Build history of the part. All positions in model axes, mm. Face numbers are marked on the shaded views. Give positions to 0.01 mm unless a question says otherwise; leave off trailing zeros. Order: outer loops, then holes, each group sorted by start corner. A loop starts at its lowest first (then second) coordinate and runs counter-clockwise, first axis right, second up. Notation, with made-up numbers: M 57.25,14.5 L 62.25,14.5 A16 ccw 62.25,41.5 Z; hole C 36,-4.75 d2. An arc over 180 degrees is marked long. One line per item, written item: value. Start each with the question number.
Autodesk Inventor part; units mm, degrees
ref_plane "YZ Plane" through (0, 0, 0) normal (1, 0, 0) x (0, 1, 0)
ref_plane "XZ Plane" through (0, 0, 0) normal (0, 1, 0) x (-1, 0, 0)
ref_plane "XY Plane" through (0, 0, 0) normal (0, 0, 1) x (1, 0, 0)
sketch "Sketch1" plane through (0, 0, 0) normal (0, 0, 1) x (1, 0, 0)
  circle A0 centre (0, 0) radius 3.9688
  dimension "d0" = 7.9375
extrude "Extrusion1" add sketch "Sketch1" along normal blind 78
thread "Thread1"
sketch "Sketch2" plane through (0, 0, 78) normal (0, 0, 1) x (1, 0, 0)
  circle A0 centre (0, 0) radius 3.9687
hole "Hole1" at (0, 0, 78) direction (0, 0, -1) diameter 6 depth 40 tip angle 118
sketch "Sketch3" plane through (0, 0, 0) normal (0, 1, 0) x (-1, 0, 0)
  line L0 (-3.9688, 78) -> (3.9688, 78)
  line L1 (-3.9688, 0) -> (3.9688, 0)
  line L2 (-1.8048, 78) -> (3.9688, 68)
  line L3 (3.9688, 0) -> (3.9688, 78)
  line L4 (-3.9688, 0) -> (-3.9688, 78)
  point P0 (0, 0)
  dimension "d12" = 30
  dimension "d13" = 10
extrude "Extrusion2" cut sketch "Sketch3" along normal mid plane 20 contours L0 L3 L2
chamfer "Chamfer1" distance 1 angle 45 1 edges at (-3.9688, 0, 0)
properties part number "ESCAPAMENTO(16)" material "Carbon Steel"
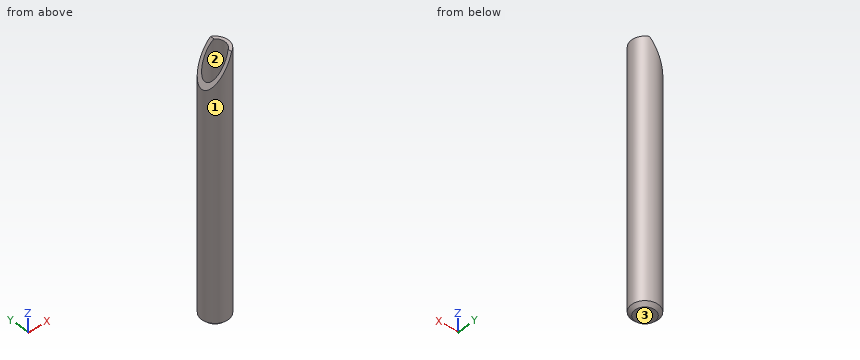
1) Drop flat-ended pins along their axis: P1, Ø3.5, axis at x = 0, y = 0, coming from the +Z side; P2, Ø1, axis at y = -2, z = 22.5, coming from the +X side. Give the stop position or say it passes through.
2) Pull direction Y, two halves, no side cores. Call the marked faces 1, 2 and 3: pulls with the +Y half, pulls with the -Y half, needs draft (parallel to the pull), parting line crosses it, or undercut.
3) Slice it at A-A (z = 42.5). List the corners of the cut face in (x, y).
4) Slice it at B-B (z = 25). List the corners of the cut face in (x, y), plus the area to 3 significant figures.
Results list:
1. P1: stops at z = 37.25
1. P2: stops at x = 3.67
2. face 1: parting line crosses it
2. face 2: undercut
2. face 3: needs draft
3. outline: C 0,0 d7.94; hole C 0,0 d6
4. outline: C 0,0 d7.94
4. area: 49.5 mm²
